Input: part model. Units: mm. Frame: model coordinates. A direction names the side the tool comes from. Give positions to 0.01 mm unless a question says otherwise; leave off trailing zeros. Order: outer loops, then holes, each group sorted by start corner. A loop starts at its lowest first (then second) coordinate and runs counter-clockwise, first axis right, second up. Notation, with made-up numbers: (30, -32.5) - (67, -32.5) arc R24 ccw to (67, -3.5) - close; hole circle Ø11 at (19.25, 11). An arc over 180 degrees is marked (long way). Use a Markdown table: item, result.
from build123d import *

# Parameters (mm, degrees)
SKETCH1_W           = 44
SKETCH1_H           = 44
SKETCH1_W_2         = 25
SKETCH1_H_2         = 40
BOSS_EXTRUDE4_DEPTH = 20
SKETCH4_W           = 44
SKETCH4_H           = 44
BOSS_EXTRUDE5_DEPTH = 2
SKETCH5_R           = 3.45
CUT_EXTRUDE2_DEPTH  = 2
SKETCH6_R           = 1.75
CUT_EXTRUDE3_DEPTH  = 23
SKETCH7_R           = 3.25
CUT_EXTRUDE4_DEPTH  = 20.5
SKETCH10_W          = 7.5
SKETCH10_H          = 25
CUT_EXTRUDE5_DEPTH  = 20
CUT_EXTRUDE6_REACH  = 46
SKETCH11_R          = 2.5
FILLET1_R           = 2.5


with BuildPart() as part:
    # Sketch1 → Boss-Extrude4 (new body)
    with BuildSketch(Plane(origin=(0, 0, 0), x_dir=(1, 0, 0), z_dir=(0, 1, 0))):
        Rectangle(SKETCH1_W, SKETCH1_H)
        Rectangle(SKETCH1_W_2, SKETCH1_H_2, mode=Mode.SUBTRACT)
    extrude(amount=BOSS_EXTRUDE4_DEPTH)

    # Sketch4 → Boss-Extrude5 (add)
    with BuildSketch(Plane.XZ):
        Rectangle(SKETCH4_W, SKETCH4_H)
    extrude(amount=BOSS_EXTRUDE5_DEPTH)

    # Sketch5 → Cut-Extrude2 (cut)
    with BuildSketch(Plane(origin=(0, 0, 0), x_dir=(1, 0, 0), z_dir=(0, 1, 0))):
        Circle(SKETCH5_R)
        with BuildLine():
            Line((-4.388708392, -8.222009531), (-1.963213799, -9.153124979))
            ThreePointArc((-1.963213799, -9.153124979), (-2.369591464, -6.58702732), (-4.388708392, -8.222009531))
        make_face()
    extrude(amount=-CUT_EXTRUDE2_DEPTH, mode=Mode.SUBTRACT)

    # Sketch6 → Cut-Extrude3 (cut, through all)
    with BuildSketch(Plane(origin=(0, 20, 0), x_dir=(1, 0, 0), z_dir=(0, 1, 0))):
        with Locations((-17.25, 17.25)):
            Circle(SKETCH6_R)
        with Locations((-17.25, -17.25)):
            Circle(SKETCH6_R)
    cut_extrude3 = extrude(amount=-CUT_EXTRUDE3_DEPTH, mode=Mode.SUBTRACT)

    # Mirror1: Cut-Extrude3 across plane
    add(cut_extrude3.mirror(Plane(origin=(0, 0, 0), x_dir=(0, 0, 1), z_dir=(1, 0, 0))), mode=Mode.SUBTRACT)

    # Sketch7 → Cut-Extrude4 (cut)
    with BuildSketch(Plane.XZ.offset(2)):
        with Locations((-17.25, 17.25)):
            Circle(SKETCH7_R)
        with Locations((17.25, 17.25)):
            Circle(SKETCH7_R)
        with Locations((17.25, -17.25)):
            Circle(SKETCH7_R)
        with Locations((-17.25, -17.25)):
            Circle(SKETCH7_R)
    extrude(amount=-CUT_EXTRUDE4_DEPTH, mode=Mode.SUBTRACT)

    # Sketch10 → Cut-Extrude5 (cut)
    with BuildSketch(Plane(origin=(0, 20, 0), x_dir=(1, 0, 0), z_dir=(0, 1, 0))):
        with Locations((-16.25, 0)):
            Rectangle(SKETCH10_W, SKETCH10_H)
    cut_extrude5 = extrude(amount=-CUT_EXTRUDE5_DEPTH, mode=Mode.SUBTRACT)

    # Mirror2: Cut-Extrude5 across plane
    add(cut_extrude5.mirror(Plane(origin=(0, 0, 0), x_dir=(0, 0, 1), z_dir=(1, 0, 0))), mode=Mode.SUBTRACT)

    # Sketch11 → Cut-Extrude6 (cut, up to next)
    with BuildSketch(Plane.XY.offset(22), mode=Mode.PRIVATE) as cut_extrude6_sk1:
        with Locations((0, 9)):
            Circle(SKETCH11_R)
    cut_extrude6_tool1 = extrude(cut_extrude6_sk1.sketch, amount=-CUT_EXTRUDE6_REACH, mode=Mode.PRIVATE) & part.part
    add(cut_extrude6_tool1.solids().sort_by_distance((0, 9, 22))[0], mode=Mode.SUBTRACT)

    # Fillet1
    fillet1_edges = [part.edges().sort_by_distance(p)[0] for p in [
        (-12.5, 10, 12.5),
        (-12.5, 10, -12.5),
        (12.5, 10, 12.5),
        (12.5, 10, -12.5),
        (22, 9, 22),
        (-22, 9, 22),
        (-22, 9, -22),
        (22, 9, -22),
    ]]
    fillet(fillet1_edges, radius=FILLET1_R)


solid = part.part
1. Section query B-B (y = 14.25). Return loops of the section in (x, z).
Response:
| item | result |
|---|---|
| outline | (-22, -19.5) arc R2.5 ccw to (-19.5, -22) - (19.5, -22) arc R2.5 ccw to (22, -19.5) - (22, 19.5) arc R2.5 ccw to (19.5, 22) - (-19.5, 22) arc R2.5 ccw to (-22, 19.5) - close; hole circle Ø6.5 at (-17.25, -17.25); hole circle Ø6.5 at (-17.25, 17.25); hole (-20, -12.5) - (-15, -12.5) arc R2.5 cw to (-12.5, -15) - (-12.5, -20) - (12.5, -20) - (12.5, -15) arc R2.5 cw to (15, -12.5) - (20, -12.5) - (20, 12.5) - (15, 12.5) arc R2.5 cw to (12.5, 15) - (12.5, 20) - (-12.5, 20) - (-12.5, 15) arc R2.5 cw to (-15, 12.5) - (-20, 12.5) - close; hole circle Ø6.5 at (17.25, -17.25); hole circle Ø6.5 at (17.25, 17.25) |
2. Section query A-A (z = -17.25). Return loops of the section in (x, y), then the cut area to 3 significant figures.
Response:
| item | result |
|---|---|
| outline | (-22, -2) - (-20.5, -2) - (-20.5, 18.5) - (-19, 18.5) - (-19, 20) - (-22, 20) - close; (-15.5, 18.5) - (-14, 18.5) - (-14, -2) - (14, -2) - (14, 18.5) - (15.5, 18.5) - (15.5, 20) - (12.5, 20) - (12.5, 0) - (-12.5, 0) - (-12.5, 20) - (-15.5, 20) - close; (19, 18.5) - (20.5, 18.5) - (20.5, -2) - (22, -2) - (22, 20) - (19, 20) - close |
| area | 191 mm^2 |
3. Section query D-D (z = -11). Return loops of the section in (x, y).
Response:
| item | result |
|---|---|
| outline | (-22, -2) - (22, -2) - (22, 20) - (20, 20) - (20, 0) - (-20, 0) - (-20, 20) - (-22, 20) - close |
4. Material intervals for line 1 along Z through (x, y) = (17.25, 19.2); line 2 along X through (y, z) = (15.5, -1.5), sorted ascending.
Response:
| item | result |
|---|---|
| line 1 | z = -22 to -19, -15.5 to -12.5, 12.5 to 15.5, 19 to 22 |
| line 2 | x = -22 to -20, 20 to 22 |
5. Pin query (flat end, axial travel): pin 1 (4 mm diameter, centred on x = 2, z = 17, fed in from +Y); pin 2 (6 mm diameter, centred on x = 17.25, z = 17.25, fed in from -Y). Return the tip coordinate at first contact, or that it passes through.
Response:
| item | result |
|---|---|
| pin 1 | stops at y = 0 |
| pin 2 | stops at y = 18.5 |
6. Section query C-C (x = -17.25). Return loops of the section in (y, z).
Response:
| item | result |
|---|---|
| outline | (-2, -22) - (20, -22) - (20, -19) - (18.5, -19) - (18.5, -20.5) - (-2, -20.5) - close; (-2, -14) - (18.5, -14) - (18.5, -15.5) - (20, -15.5) - (20, -12.5) - (0, -12.5) - (0, 12.5) - (20, 12.5) - (20, 15.5) - (18.5, 15.5) - (18.5, 14) - (-2, 14) - close; (-2, 20.5) - (18.5, 20.5) - (18.5, 19) - (20, 19) - (20, 22) - (-2, 22) - close |
7. Set-up query: faces 4 (the face through (18, 10, 12.5)), 5 (the face through (-19.645, 8.107, 19.447)), 6 (the face through (-3.193, -0.986, 8.681)), 7 (the face through (-0.54, 6.56, 21.01)). Return all of +Z, -Z, +X, -X, +Y, -Y with unobstructed straight access to the full face (end or side cutting, diameter ignored); none if empty.
Response:
| item | result |
|---|---|
| face 4 | +Y |
| face 5 | -Y |
| face 6 | +Y, -Y |
| face 7 | +Z |
8. Mould query, pull axis X, two halves, no side actions, for faces 1 (the face through (-21.287, 8.846, -21.248)), 2 (the face through (17.478, 19.26, -18.985)), 3 (the face through (21.248, 9.154, 21.287)). Classes: pulls with the +X half, pulls with the -X half, needs draft (parallel to the pull), parting line crosses it, or undercut.
Response:
| item | result |
|---|---|
| face 1 | pulls with the -X half |
| face 2 | undercut |
| face 3 | pulls with the +X half |
